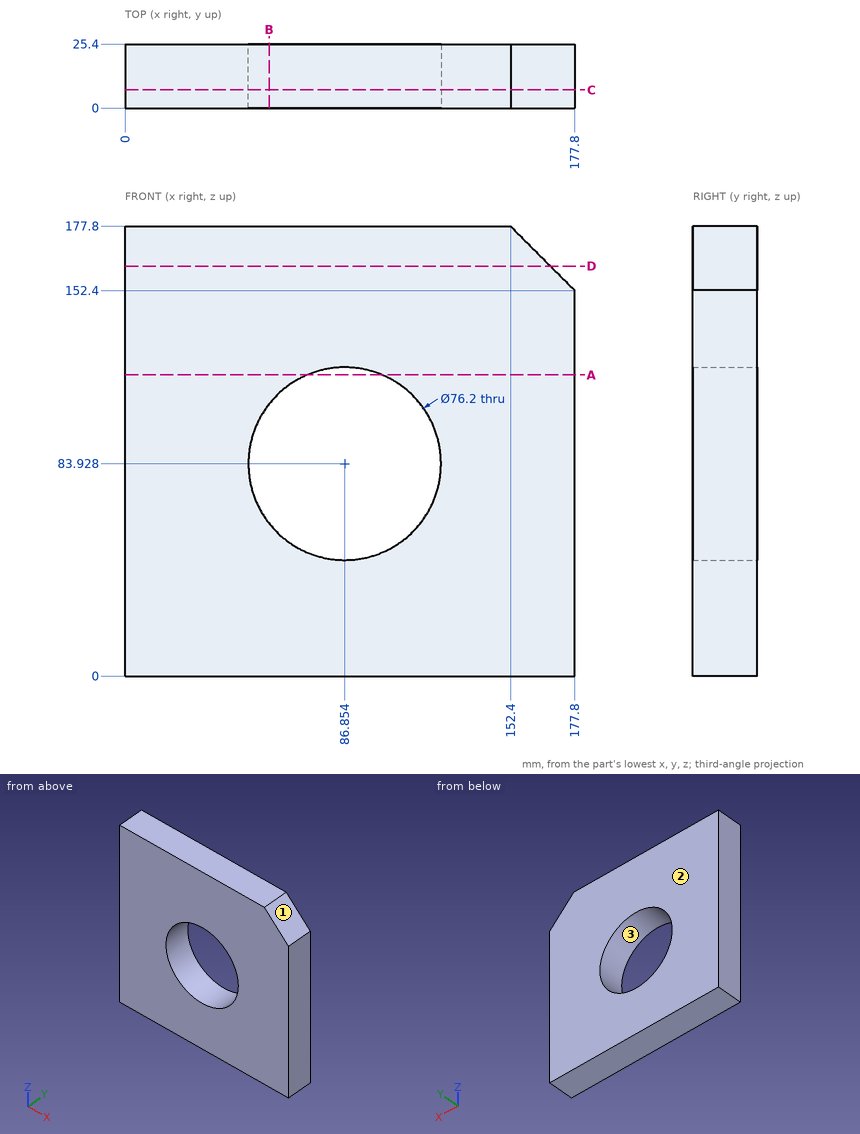
For this review, use the dimensioned drawing (mm, ordinates from the lowest corner) and the shaded views. Round coordinates to 2 decimals unless told otherwise and drop trailing zeros. Write each loop counter-clockwise with the first axis right and the second up, starting at its lowest first coordinate (ties: lowest second). Pieces come first, ordered by that corner, then holes. Notation, with made-up numbers: M 87.25,27.5 L 118.25,27.5 A35 ccw 118.25,66.5 Z; hole C 70.5,89.5 d8. An arc over 180 degrees is marked long. Write item = value, one per line. Start each with the question number.
(1) We need section A-A (z = 119). Give the boundary of the cut face in (x, y).
(2) The part is to be moulded in two halves that separate along Z. For the marked faces 1, 2 and 3, say which applies: +Z half, -Z half, draft (parallel to the pull), parting line (faces both ways), or undercut.
(3) We need section C-C (y = 7.25). Give the boundary of the cut face in (x, z), then the cut area to 3 significant figures.
(4) For line 1 along X through (y, z) = (10.5, 84); line 2 along X through (y, z) = (8.75, 56) (1 decimal); line 3 along Z through (x, y) = (82.5, 3.5), list the stretches that pass through material, from the lowest coordinate up.
(5) We need section D-D (z = 162). Give the boundary of the cut face in (x, y), then the cut area to 3 significant figures.
(6) We need section B-B (x = 57). Give the boundary of the cut face in (y, z) (1 decimal).
Results found:
q1.outline = M 0,0 L 71.97,0 L 71.97,25.4 L 0,25.4 Z; M 101.74,0 L 177.8,0 L 177.8,25.4 L 101.74,25.4 Z
q2.face_1 = +Z half
q2.face_2 = draft
q2.face_3 = undercut
q3.outline = M 0,0 L 177.8,0 L 177.8,152.4 L 152.4,177.8 L 0,177.8 Z; hole C 86.85,83.93 d76.2
q3.area = 26,700 mm²
q4.line_1 = 0 to 48.75, 124.95 to 177.8
q4.line_2 = 0 to 60.9, 112.8 to 177.8
q4.line_3 = 0 to 46.08, 121.78 to 177.8
q5.outline = M 0,0 L 168.2,0 L 168.2,25.4 L 0,25.4 Z
q5.area = 4,270 mm²
q6.outline = M 0,0 L 25.4,0 L 25.4,60.3 L 0,60.3 Z; M 0,107.6 L 25.4,107.6 L 25.4,177.8 L 0,177.8 Z
